from build123d import *

# Parameters (mm, degrees)
SKETCH1_W           = 99.9236
SKETCH1_H           = 45.085
BOSS_EXTRUDE1_DEPTH = 19.304
SKETCH2_W           = 120.8278
SKETCH2_H           = 45.085
BOSS_EXTRUDE2_DEPTH = 1.016
SKETCH3_W           = 86.580193544
SKETCH3_H           = 5.780372674
CUT_EXTRUDE1_DEPTH  = 5


with BuildPart() as part:
    # Sketch1 → Boss-Extrude1 (new body)
    with BuildSketch(Plane(origin=(0, 0, 0), x_dir=(1, 0, 0), z_dir=(0, 1, 0))):
        with Locations((49.9618, 22.5425)):
            Rectangle(SKETCH1_W, SKETCH1_H)
    extrude(amount=BOSS_EXTRUDE1_DEPTH)

    # Sketch2 → Boss-Extrude2 (add)
    with BuildSketch(Plane.XZ):
        with Locations((49.9618, -22.5425)):
            Rectangle(SKETCH2_W, SKETCH2_H)
        with BuildLine():
            Line((-3.7973, -9.1567), (-3.7973, -10.7823))
            ThreePointArc((-3.7973, -10.7823), (-5.588, -12.573), (-7.3787, -10.7823))
            Line((-7.3787, -10.7823), (-7.3787, -9.1567))
            ThreePointArc((-7.3787, -9.1567), (-5.588, -7.366), (-3.7973, -9.1567))
        make_face(mode=Mode.SUBTRACT)
        with BuildLine():
            Line((-3.7973, -35.9283), (-3.7973, -34.3027))
            ThreePointArc((-3.7973, -34.3027), (-5.588, -32.512), (-7.3787, -34.3027))
            Line((-7.3787, -34.3027), (-7.3787, -35.9283))
            ThreePointArc((-7.3787, -35.9283), (-5.588, -37.719), (-3.7973, -35.9283))
        make_face(mode=Mode.SUBTRACT)
        with BuildLine():
            Line((103.7209, -9.1567), (103.7209, -10.7823))
            ThreePointArc((103.7209, -10.7823), (105.5116, -12.573), (107.3023, -10.7823))
            Line((107.3023, -10.7823), (107.3023, -9.1567))
            ThreePointArc((107.3023, -9.1567), (105.5116, -7.366), (103.7209, -9.1567))
        make_face(mode=Mode.SUBTRACT)
        with BuildLine():
            Line((103.7209, -35.9283), (103.7209, -34.3027))
            ThreePointArc((103.7209, -34.3027), (105.5116, -32.512), (107.3023, -34.3027))
            Line((107.3023, -34.3027), (107.3023, -35.9283))
            ThreePointArc((107.3023, -35.9283), (105.5116, -37.719), (103.7209, -35.9283))
        make_face(mode=Mode.SUBTRACT)
    extrude(amount=BOSS_EXTRUDE2_DEPTH)

    # Sketch3 → Cut-Extrude1 (cut)
    with BuildSketch(Plane(origin=(0, 0, -45.085), x_dir=(-1, 0, 0), z_dir=(0, 0, -1))):
        with Locations((-49.9618, 9.652)):
            Rectangle(SKETCH3_W, SKETCH3_H)
    extrude(amount=-CUT_EXTRUDE1_DEPTH, mode=Mode.SUBTRACT)


solid = part.part
Verification items for the finished model (mm, model axes). A direction names the side the tool comes from. Give positions to 0.01 mm unless a question says otherwise; leave off trailing zeros. Write each loop counter-clockwise with the first axis right and the second up, starting at its lowest first coordinate (ties: lowest second). Pieces come first, ordered by that corner, then holes. Notation, with made-up numbers: (70.5, 45) -> (122.5, 45) arc R21 cw to (122.5, 57) -> close; hole circle Ø7 at (33.5, 9). An arc over 180 degrees is marked (long way). Use CSV: the item, a comma, the result in double quotes.
(1) Release check for a two-part mould opening along Y. For faces 5 (the flat face through (51, 6.762, -43)), 6 (the flat face through (49, 19.304, -23)), 7 (the flat face through (49, -1.016, -22)) record: +Y half, -Y half, draft (parallel to the pull), parting line (faces both ways), or undercut.
Derived:
face 5,"undercut"
face 6,"+Y half"
face 7,"-Y half"
(2) Sectioned sample at C-C (y = 15.5). Record the cut outline in (x, z) (3 decimals).
Derived:
outline,"(0, -45.085) -> (99.924, -45.085) -> (99.924, 0) -> (0, 0) -> close"
(3) Go/stop test with flat-tipped pins: pin 1 (11.5 mm diameter, centred on x = 107, z = -18.5, fed in from +Y); pin 2 (4 mm diameter, centred on y = 8.5, z = -43, fed in from -X); pin 3 (2 mm diameter, centred on x = 46.5, y = 4.5, fed in from +Z); pin 4 (3 mm diameter, centred on x = 53, y = 10.5, fed in from -Z) (3 decimals). Record where each tip stops, or that it passes through.
Derived:
pin 1,"stops at y = 0"
pin 2,"stops at x = 0"
pin 3,"stops at z = 0"
pin 4,"stops at z = -40.085"
(4) Set-up check for faces 1 (the flat face through (105, 0, -22)), 2 (the flat face through (49, 9, 0)), 3 (the flat face through (0, 10, -22)), 4 (the flat face through (51, 12.542, -43)): record each of +Z, -Z, +X, -X, +Y, -Y from which the full face is reachable in a straight line by a thin tool's end or side.
Derived:
face 1,"+Z, -Z, +X, +Y"
face 2,"+Z, +X, -X, +Y, -Y"
face 3,"+Z, -Z, -X, +Y"
face 4,"-Z"
(5) Material ranges on L1, parallel to X at y = 5.75, z = -11; L2, parallel to Y at x = 50, z = -43; L3, parallel to Z at x = 30.5, y = 9.25 (3 decimals), recorded low to high.
Derived:
L1,"x = 0 to 99.92"
L2,"y = -1.02 to 6.76, 12.54 to 19.3"
L3,"z = -40.085 to 0"
(6) Sectioned sample at A-A (x = 63). Record the cut outline in (y, z) (3 decimals), plus the area to 3 significant figures.
Derived:
outline,"(-1.016, -45.085) -> (6.762, -45.085) -> (6.762, -40.085) -> (12.542, -40.085) -> (12.542, -45.085) -> (19.304, -45.085) -> (19.304, 0) -> (-1.016, 0) -> close"
area,"887 mm^2"
(7) Sectioned sample at B-B (z = -30). Record the cut outline in (x, y).
Derived:
outline,"(-10.45, -1.02) -> (110.38, -1.02) -> (110.38, 0) -> (99.92, 0) -> (99.92, 19.3) -> (0, 19.3) -> (0, 0) -> (-10.45, 0) -> close"
